Read the model definition and answer for the solid it produces. Units are mm, in the model's axes. Coordinates: 2 decimals unless noted, no trailing zeros. Write each loop counter-clockwise with the first axis right and the second up, starting at its lowest first coordinate (ties: lowest second). Pieces come first, ordered by that corner, then holes. Notation, with made-up numbers: (-6, -11.75) -> (24, -11.75) arc R32 ccw to (24, 21.25) -> close; hole circle Ø7 at (10.5, -16). An arc over 180 degrees is marked (long way). Answer as a JSON object with one key per item and string values. Group by question number.
(1) Find section D-D (z = 4.25). Give the vertices of the cut face in (x, y), then the cut area to 3 significant figures.
(2) Find section C-C (x = 0). Give the vertices of the cut face in (y, z), then the cut area to 3 significant figures.
(3) Flat-ended cylindrical pins translate along their axes: P1, Ø4, axis at x = 37.5, z = 5.5, coming from the +Y side; P2, Ø1, axis at y = 21.5, z = 11.5, coming from the +X side; P3, Ø10, axis at x = 24.5, y = -2.5, coming from the -Z side. Find the tip coordinate at first contact, or state that the pin passes through.
(4) Straight lines are drawn through the part: L1, parallel to Y at x = 0, z = 9.25; L2, parallel to Y at x = -22, z = 1.25; L3, parallel to X at y = 0.5, z = 6.5. For each, find the intervals that lie inside material, in ascending order.
(5) Find section B-B (x = 16.5). Give the vertices of the cut face in (y, z), then the cut area to 3 significant figures.
(6) For a pull along Z with two mould halves and no side action, classify faces 1 (the face through (5.257, -29.127, 5.513)), 2 (the face through (-23, 8, 0)), 3 (the face through (-23, 8, 12.7)), 4 (the face through (-50, 0, 6)) as +Z half, -Z half, draft (parallel to the pull), parting line (faces both ways), or undercut.
(7) Find section A-A (y = 0). Give the vertices of the cut face in (x, z).
from build123d import *

# Parameters (mm, degrees)
F0_W     = 100
F0_H     = 70
F0_R     = 24
F1_DEPTH = 12.7
F2_R     = 25.4
F4_D     = 8
F4_DEPTH = 12.7


with BuildPart() as f1:
    # F0 (on Top) → F1 (new body)
    with BuildSketch(Plane.XY):
        Rectangle(F0_W, F0_H)
        Circle(F0_R, mode=Mode.SUBTRACT)
    extrude(amount=F1_DEPTH)

    # F2
    f2_edges = [f1.edges().sort_by_distance(p)[0] for p in [
        (50, -35, 6.35),
        (50, 35, 6.35),
    ]]
    fillet(f2_edges, radius=F2_R)

    # F4
    with Locations(Plane.XZ.offset(35)):
        with Locations((1.260702, 5.33683)):
            Hole(F4_D / 2, depth=F4_DEPTH)


solid = f1.part
Results below:
{
 "1": {"outline": "(-50, -35) -> (-2.59, -35) -> (-2.59, -23.86) arc R24 cw (long way) to (5.11, -23.45) -> (5.11, -35) -> (24.6, -35) arc R25.4 ccw to (50, -9.6) -> (50, 9.6) arc R25.4 ccw to (24.6, 35) -> (-50, 35) -> close", "area": "4,830 mm2"},
 "2": {"outline": "(-35, 0) -> (-24, 0) -> (-24, 1.54) -> (-35, 1.54) -> close; (-35, 9.13) -> (-24, 9.13) -> (-24, 12.7) -> (-35, 12.7) -> close; (24, 0) -> (35, 0) -> (35, 12.7) -> (24, 12.7) -> close", "area": "196 mm2"},
 "3": {"P1": "stops at y = 32.54", "P2": "stops at x = 47.3", "P3": "stops at z = 0"},
 "4": {"L1": "y = -35 to -24, 24 to 35", "L2": "y = -35 to -9.59, 9.59 to 35", "L3": "x = -50 to -23.99, 23.99 to 50"},
 "5": {"outline": "(-35, 0) -> (-17.43, 0) -> (-17.43, 12.7) -> (-35, 12.7) -> close; (17.43, 0) -> (35, 0) -> (35, 12.7) -> (17.43, 12.7) -> close", "area": "446 mm2"},
 "6": {"face 1": "undercut", "face 2": "-Z half", "face 3": "+Z half", "face 4": "draft"},
 "7": {"outline": "(-50, 0) -> (-24, 0) -> (-24, 12.7) -> (-50, 12.7) -> close; (24, 0) -> (50, 0) -> (50, 12.7) -> (24, 12.7) -> close"}
}
